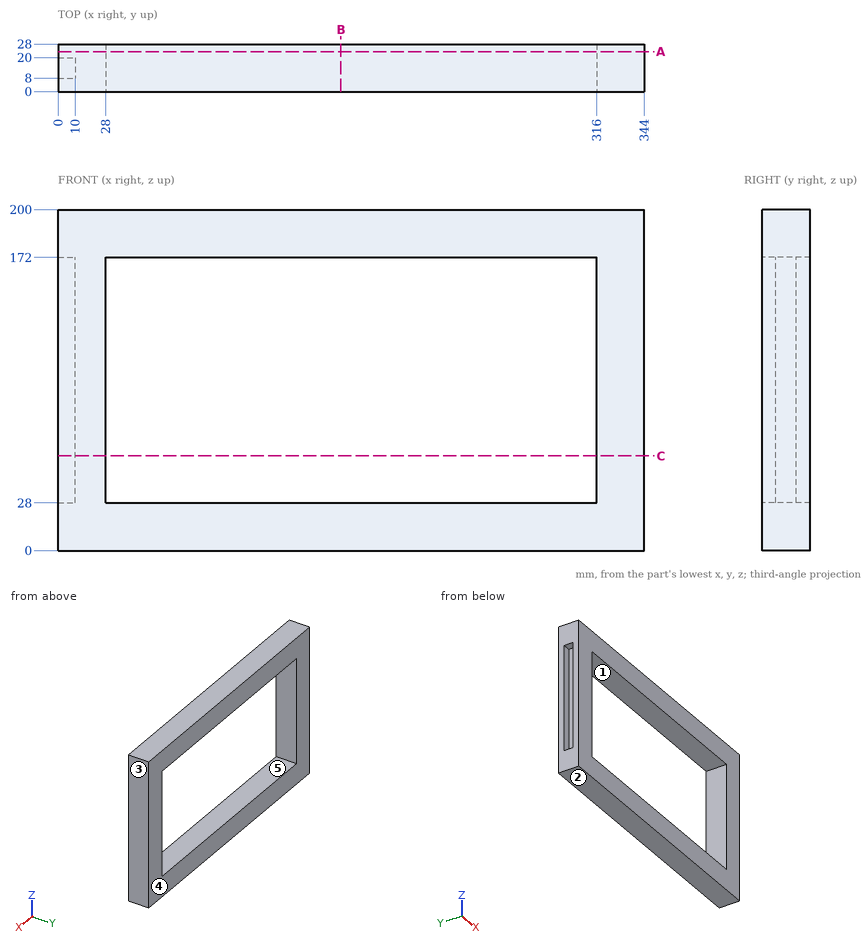
Verification items for this drawing (mm, ordinates from the low corner). A direction names the side the tool comes from. Give positions to 0.01 mm unless a question says otherwise; leave off trailing zeros. Loops run counter-clockwise (first coordinate to the right, second up) from the corner with the lowest first, then second, coordinate; pieces in that order, holes last. Notation, with made-up numbers: M 13.25,-37 L 63.25,-37 A10 ccw 63.25,-33 Z; hole C 12,75.25 d3. An arc over 180 degrees is marked long. Return JSON: item names as keys, results as strings. Group by question number.
1. Cross-section at C-C on z = 55.5. Record the boundary of the cut face in (x, y), plus the area to 3 significant figures.
2. Cross-section at A-A on y = 23.5. Record the boundary of the cut face in (x, z).
3. Go/stop test with a flat-tipped pin: pin 1 (3.5 mm diameter, centred on y = 12, z = 91, fed in from -X). Record where the tip stops, or that it passes through.
4. Thickness scan on L1, parallel to Z at x = 121, y = 12.5; L2, parallel to X at y = 21, z = 127.5; L3, parallel to X at y = 14.25, z = 70. Record the ranges inside material, lowest first.
5. Mould release check, pull along X, two halves, no side actions. Record for the marked faces 3, 4 and 5: released by +X, released by -X, zero draft, split by the parting line, or undercut.
6. Cross-section at B-B on x = 166. Record the boundary of the cut face in (y, z).
7. Tool access check on the marked faces 1 and 2. Record the directions out of +Z, -Z, +X, -X, +Y, -Y that give a thin tool (end or side, any length) a straight path to the whole face; none if there is none.
Return value:
{
 "1": {"outline": "M 0,0 L 28,0 L 28,28 L 0,28 L 0,20 L 10,20 L 10,8 L 0,8 Z; M 316,0 L 344,0 L 344,28 L 316,28 Z", "area": "1,450 mm^2"},
 "2": {"outline": "M 0,0 L 344,0 L 344,200 L 0,200 Z; hole M 28,28 L 316,28 L 316,172 L 28,172 Z"},
 "3": {"pin 1": "x = 10"},
 "4": {"L1": "0 to 28, 172 to 200", "L2": "0 to 28, 316 to 344", "L3": "10 to 28, 316 to 344"},
 "5": {"face 3": "released by +X", "face 4": "zero draft", "face 5": "undercut"},
 "6": {"outline": "M 0,0 L 28,0 L 28,28 L 0,28 Z; M 0,172 L 28,172 L 28,200 L 0,200 Z"},
 "7": {"face 1": "+Y, -Y", "face 2": "-Z, +X, -X, +Y, -Y"}
}
